from build123d import *

# Parameters (mm, degrees)
SKETCH_1_R              = 11.25
EXTRUDE_1_DEPTH         = 13
SKETCH_2_W              = 20
SKETCH_2_H              = 20
CUT_EXTRUDE_1_DEPTH     = 127.393235578
CUT_EXTRUDE1_DEPTH      = 75.399260749
CUT_EXTRUDE1_DEPTH_BACK = 75.399260749
SKETCH1_R               = 2.75


with BuildPart() as part:
    # Эскиз1 → Бобышка-Вытянуть1 (new, symmetric)
    with BuildSketch(Plane(origin=(0, 0, 0), x_dir=(1, 0, 0), z_dir=(0, 1, 0))):
        Polygon((-60, -10.5), (60, -10.5), (60, 10.5), (50.172803675, 37.5), (0, 37.5), (-50.172803675, 37.5), (-60, 10.5), align=None)
        with Locations(Location((0, 23.5, 0), (0, 0, 90))):
            Circle(SKETCH_1_R, mode=Mode.SUBTRACT)
        with Locations(Location((-40, 23.5, 0), (0, 0, 90))):
            Circle(SKETCH_1_R, mode=Mode.SUBTRACT)
        with Locations(Location((40, 23.5, 0), (0, 0, 90))):
            Circle(SKETCH_1_R, mode=Mode.SUBTRACT)
    extrude(amount=EXTRUDE_1_DEPTH, both=True)

    # Эскиз2 → Вырез-Вытянуть1 (cut, through all)
    with BuildSketch(Plane.ZY.offset(60)):
        with Locations((0.5, 0)):
            Rectangle(SKETCH_2_W, SKETCH_2_H)
    extrude(amount=-CUT_EXTRUDE_1_DEPTH, mode=Mode.SUBTRACT)

    # Sketch1 → Cut-Extrude1 (cut, two sides: drawn at the far end of the back side and taken through both)
    with BuildSketch(Plane.XZ.offset(-10).offset(-CUT_EXTRUDE1_DEPTH_BACK)):
        with Locations(Location((45, 0.5, 0), (0, 0, 270))):
            Circle(SKETCH1_R)
        with Locations(Location((-45, 0.5, 0), (0, 0, 270))):
            Circle(SKETCH1_R)
    extrude(amount=CUT_EXTRUDE1_DEPTH + CUT_EXTRUDE1_DEPTH_BACK, mode=Mode.SUBTRACT)


solid = part.part
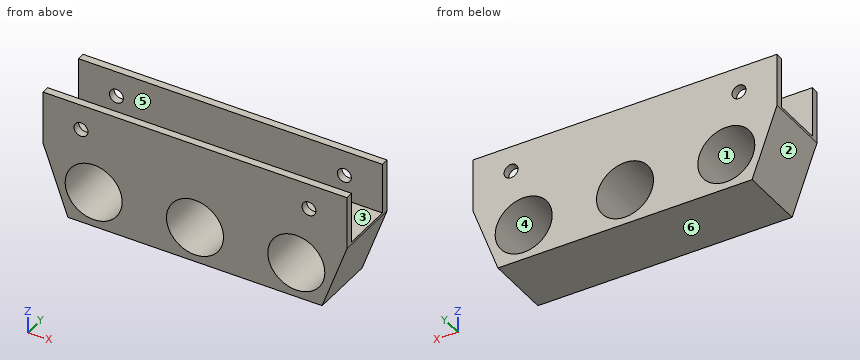
Here's how the part is built. I have some questions about the finished solid (model axes, mm). Face numbers are marked on the shaded views. A direction names the side the tool comes from. Coordinates: 2 decimals unless noted, no trailing zeros. Order: outer loops, then holes, each group sorted by start corner. A loop starts at its lowest first (then second) coordinate and runs counter-clockwise, first axis right, second up. Notation, with made-up numbers: (25.25, -25.75) -> (76.25, -25.75) arc R19 cw to (76.25, -0.75) -> close; hole circle Ø5 at (-10.5, -33.75). An arc over 180 degrees is marked (long way). Answer in a Markdown table with one row per item.
(1) I want a section at B-B on x = 40. List the corners of the cut face in (y, z) for me, then the cut area to 3 significant figures.
Answer key:
| item | result |
|---|---|
| outline | (-13, -37.5) -> (13, -37.5) -> (13, -34.75) -> (-13, -34.75) -> close; (-13, -12.25) -> (13, -12.25) -> (13, 10.5) -> (10, 10.5) -> (10, -9.5) -> (-10, -9.5) -> (-10, 10.5) -> (-13, 10.5) -> close |
| area | 263 mm^2 |
(2) I want a section at A-A on z = 5. List the corners of the cut face in (x, y) for me, then the cut area to 3 significant figures.
Answer key:
| item | result |
|---|---|
| outline | (-60, -13) -> (60, -13) -> (60, -10) -> (-60, -10) -> close; (-60, 10) -> (60, 10) -> (60, 13) -> (-60, 13) -> close |
| area | 720 mm^2 |
(3) Will these pins go through, and if not, where does the flat tip stop? pin 1 Ø9 at (x, z) = (-45, 0.5) entering from +Y; pin 2 Ø1 at (y, z) = (-1, -32.5) entering from -X; pin 3 Ø10 at (y, z) = (7.5, -27.5) entering from -X; pin 4 Ø18 at (x, z) = (-40, -23.5) entering from -Y.
Answer key:
| item | result |
|---|---|
| pin 1 | y = 13 |
| pin 2 | x = -52.17 |
| pin 3 | x = -55.63 |
| pin 4 | through |
(4) I want a section at D-D on z = -27. List the corners of the cut face in (x, y) for me.
Answer key:
| item | result |
|---|---|
| outline | (-53.99, -13) -> (-50.69, -13) -> (-50.69, 13) -> (-53.99, 13) -> close; (-29.31, -13) -> (-10.69, -13) -> (-10.69, 13) -> (-29.31, 13) -> close; (10.69, -13) -> (29.31, -13) -> (29.31, 13) -> (10.69, 13) -> close; (50.69, -13) -> (53.99, -13) -> (53.99, 13) -> (50.69, 13) -> close |
(5) Thinking about a two-plate mould opening in X: for the marked faces 1, 2, 3 and 4, which applies, +X half, -X half, draft (parallel to the pull), parting line (faces both ways), or undercut?
Answer key:
| item | result |
|---|---|
| face 1 | undercut |
| face 2 | -X half |
| face 3 | draft |
| face 4 | undercut |
(6) On a 3-axis mill with a long thin cutter (end or side, diameter ignored), from which of +Z, -Z, +X, -X, +Y, -Y can I reach the whole of each face in a straight line? I mean the marked faces 5 and 6. Say none if no direction works.
Answer key:
| item | result |
|---|---|
| face 5 | +Z, +X, -X |
| face 6 | -Z, +X, -X, +Y, -Y |
(7) Please list where these lines run through material, in increasing order: probe 1 along X at (y, z) = (-12.05, 0.5); probe 2 along Z at (x, y) = (39.5, 2.5); probe 3 along Z at (x, y) = (-45, 11.95).
Answer key:
| item | result |
|---|---|
| probe 1 | -60 to -47.75, -42.25 to 42.25, 47.75 to 60 |
| probe 2 | -37.5 to -34.74, -12.26 to -9.5 |
| probe 3 | -37.5 to -33.58, -13.42 to -2.25, 3.25 to 10.5 |
(8) I want a section at C-C on y = 11.5. List the corners of the cut face in (x, z) for me, then the cut area to 3 significant figures.
Answer key:
| item | result |
|---|---|
| outline | (-60, -10.5) -> (-50.17, -37.5) -> (50.17, -37.5) -> (60, -10.5) -> (60, 10.5) -> (-60, 10.5) -> close; hole circle Ø22.5 at (-40, -23.5); hole circle Ø5.5 at (-45, 0.5); hole circle Ø22.5 at (0, -23.5); hole circle Ø22.5 at (40, -23.5); hole circle Ø5.5 at (45, 0.5) |
| area | 4,250 mm^2 |
